Geometry: see drawing. Coordinates: mm, zero at the bounding-box minimum. A direction names the side the tool comes from. Round coordinates to 2 decimals unless told otherwise and drop trailing zeros. Loops run counter-clockwise (first coordinate to the right, second up) from the corner with the lowest first, then second, coordinate; pieces in that order, holes last. Notation, with made-up numbers: (74.25, 7.5) - (91.25, 7.5) arc R9 cw to (91.25, 11.5) - close; hole circle Ø9 at (3, -29). An arc over 180 degrees is marked (long way). Use CSV: the item, a comma, the result in double quotes.
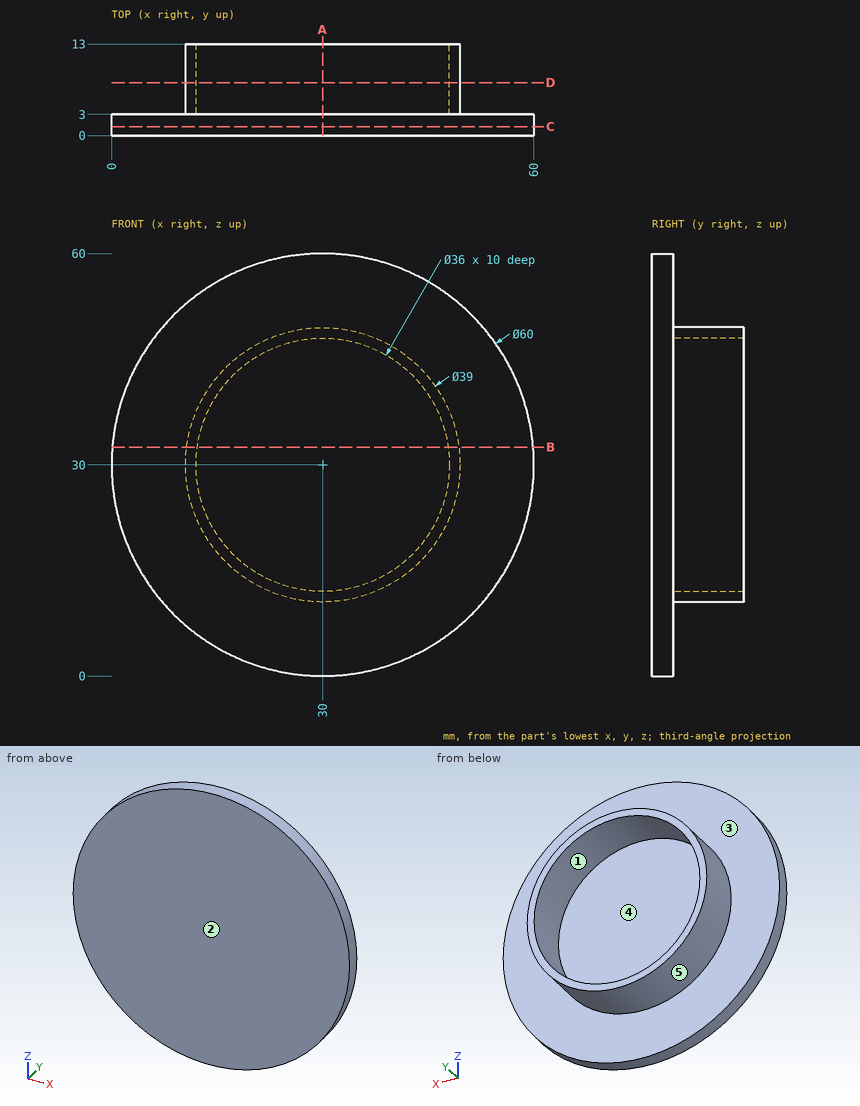
Item 1: Mould query, pull axis X, two halves, no side actions, for the marked faces 3, 4 and 5. Classes: released by +X, released by -X, zero draft, split by the parting line, or undercut.
Final values:
face 3,"zero draft"
face 4,"undercut"
face 5,"split by the parting line"
Item 2: Reachability of the marked faces 1 and 2 from +Z, -Z, +X, -X, +Y, -Y: full face, straight path, thin tool, end or side. Return the list, or none.
Final values:
face 1,"+Y"
face 2,"+Z, -Z, +X, -X, -Y"
Item 3: Section A-A on x = 30. Return the cut outline in (y, z), plus the area to 3 significant figures.
Final values:
outline,"(0, 0) - (3, 0) - (3, 10.5) - (13, 10.5) - (13, 12) - (3, 12) - (3, 48) - (13, 48) - (13, 49.5) - (3, 49.5) - (3, 60) - (0, 60) - close"
area,"210 mm²"
Item 4: Section C-C on y = 1.25. Return the cut outline in (x, z).
Final values:
outline,"circle Ø60 at (30, 30)"
Item 5: Pin query (flat end, axial travel): P1, Ø6, axis at x = 16, y = 4, coming from the -Z side; P2, Ø4, axis at x = 36, y = 7.5, coming from the -Z side; P3, Ø18, axis at x = 26.5, z = 31, coming from the +Y side. Return the tip coordinate at first contact, or that it passes through.
Final values:
P1,"stops at z = 2.16"
P2,"stops at z = 10.91"
P3,"stops at y = 3"
Item 6: Material intervals for line 1 (Z direction, x = 30, y = 7.75); line 2 (Y direction, x = 14, z = 10), sorted ascending.
Final values:
line 1,"z = 10.5 to 12, 48 to 49.5"
line 2,"y = 0 to 3"
Item 7: Section B-B on z = 32.5. Return the cut outline in (x, y).
Final values:
outline,"(0.1, 0) - (59.9, 0) - (59.9, 3) - (49.34, 3) - (49.34, 13) - (47.83, 13) - (47.83, 3) - (12.17, 3) - (12.17, 13) - (10.66, 13) - (10.66, 3) - (0.1, 3) - close"
Item 8: Section D-D on y = 7.5. Return the cut outline in (x, z), plus the area to 3 significant figures.
Final values:
outline,"circle Ø39 at (30, 30); hole circle Ø36 at (30, 30)"
area,"177 mm²"
